from build123d import *

# Parameters (mm, degrees)
BOSS_EXTRUDE1_DEPTH   = 63
BOSS_EXTRUDE1_2_DEPTH = 63
BOSS_EXTRUDE2_DEPTH   = 51
BOSS_EXTRUDE3_DEPTH   = 22
BOSS_EXTRUDE4_START   = 41
BOSS_EXTRUDE4_DEPTH   = 22
BOSS_EXTRUDE5_START   = 19
BOSS_EXTRUDE5_DEPTH   = 22


with BuildPart() as part:
    # Sketch1 → Boss-Extrude1 (new body)
    with BuildSketch(Plane(origin=(0, 0, 0), x_dir=(0, 0, -1), z_dir=(1, 0, 0))):
        Polygon((-75, 0), (-50, 0), (-50, 24.666666667), (-63, 18.08), (-75, 12), align=None)
    extrude(amount=BOSS_EXTRUDE1_DEPTH)



with BuildPart() as body_2:
    # Sketch1 → Boss-Extrude1 2 (new body)
    with BuildSketch(Plane(origin=(0, 0, 0), x_dir=(0, 0, -1), z_dir=(1, 0, 0))):
        Polygon((-25, 0), (0, 0), (0, 38), (-23.684210526, 38), (-25, 37.333333333), align=None)
    extrude(amount=BOSS_EXTRUDE1_2_DEPTH)


with BuildPart() as part_1:
    add(part.part)

    add(body_2.part)  # Boss-Extrude2 merges body 2
    # Sketch1_3 → Boss-Extrude2 (add)
    with BuildSketch(Plane(origin=(0, 0, 0), x_dir=(0, 0, -1), z_dir=(1, 0, 0))):
        Polygon((-50, 0), (-25, 0), (-25, 37.333333333), (-31.421052632, 34.08), (-50, 24.666666667), align=None)
    extrude(amount=BOSS_EXTRUDE2_DEPTH)

    # Sketch1_4 → Boss-Extrude3 (add)
    with BuildSketch(Plane(origin=(0, 0, 0), x_dir=(0, 0, -1), z_dir=(1, 0, 0))):
        Polygon((-23.684210526, 38), (0, 38), (0, 50), align=None)
    extrude(amount=BOSS_EXTRUDE3_DEPTH)

    # Sketch1_5 → Boss-Extrude4 (add)
    with BuildSketch(Plane(origin=(0, 0, 0), x_dir=(0, 0, -1), z_dir=(1, 0, 0)).offset(BOSS_EXTRUDE4_START)):
        Polygon((-23.684210526, 38), (0, 38), (0, 50), align=None)
    extrude(amount=BOSS_EXTRUDE4_DEPTH)

    # Sketch1_6 → Boss-Extrude5 (add)
    with BuildSketch(Plane(origin=(0, 0, 0), x_dir=(0, 0, -1), z_dir=(1, 0, 0)).offset(BOSS_EXTRUDE5_START)):
        Polygon((-63, 18.08), (-50, 24.666666667), (-31.421052632, 34.08), (-63, 34.08), align=None)
    extrude(amount=BOSS_EXTRUDE5_DEPTH)


solid = part_1.part
Read the model definition and answer for the solid it produces. Units are mm, in the model's axes. A direction names the side the tool comes from. Coordinates: 2 decimals unless noted, no trailing zeros. Loops run counter-clockwise (first coordinate to the right, second up) from the corner with the lowest first, then second, coordinate; pieces in that order, holes last.
Q1. The part is cut by section C-C on y = 40. Write down the section's boundary in (x, z).
Q2. The part is cut by section D-D on x = 58. Write down the section's boundary in (y, z), and give its area (3 significant figures).
Q3. Which of the six approach directions +Z, -Z, +X, -X, +Y, -Y give full straight-line access (tool end or side, diameter ignored) to faces 1 (the face through (57, 12, 50)), 2 (the face through (31, 38, 12)), 3 (the face through (41, 28, 51)), 4 (the face through (30, 34.08, 47)), 5 (the face through (19, 28, 51))?
Q4. Consider probe 1 along Z at (x, y) = (39.5, 25.5); probe 2 along X at (y, z) = (10.5, 29); probe 3 along Y at (x, z) = (35, 56.5). Determine where each line is inside the solid, lowest interval first.
Q5. The mould has two halves that part along Z. Classify faces 6 (the face through (51, 15, 38)), 7 (the face through (41, 41, 7)), 8 (the face through (30, 26, 63)): +Z half, -Z half, draft (parallel to the pull), parting line (faces both ways), or undercut.
Q6. The part is cut by section A-A on x = 11.5. Write down the section's boundary in (y, z), and give its area (4 significant figures).
Q7. The part is cut by section B-B on z = 15. Write down the section's boundary in (x, y), and give its area (3 significant figures).
Q8. Each of these flat-tipped pins is pushed along its axis until it touches: pin 1 Ø5 at (x, z) = (47, 29.5) entering from +Y; pin 2 Ø3 at (x, y) = (14, 31) entering from +Z; pin 3 Ø8 at (x, y) = (32, 26) entering from +Z. Where does it stop, or does it pass through?
Results below:
1. outline: (0, 0) - (22, 0) - (22, 19.74) - (0, 19.74) - close; (41, 0) - (63, 0) - (63, 19.74) - (41, 19.74) - close
2. outline: (0, 0) - (50, 0) - (37.33, 25) - (0, 25) - close; (0, 50) - (24.67, 50) - (12, 75) - (0, 75) - close
2. area: 1,550 mm2
3. face 1: +X, +Y, -Y
3. face 2: +Z, -Z, +Y
3. face 3: +Z, +X, +Y
3. face 4: +Z, +X, -X, +Y
3. face 5: +Z, -X, +Y
4. probe 1: z = 0 to 63
4. probe 2: x = 0 to 51
4. probe 3: y = 0 to 34.08
5. face 6: undercut
5. face 7: draft
5. face 8: +Z half
6. outline: (0, 0) - (50, 0) - (12, 75) - (0, 75) - close
6. area: 2,325 mm2
7. outline: (0, 0) - (63, 0) - (63, 42.4) - (41, 42.4) - (41, 38) - (22, 38) - (22, 42.4) - (0, 42.4) - close
7. area: 2,590 mm2
8. pin 1: stops at y = 36.32
8. pin 2: stops at z = 40.46
8. pin 3: stops at z = 63
